Check sheet for the modelled part. Datum: model origin and axes. Units: mm. Round coordinates to 2 decimals unless told otherwise and drop trailing zeros. Write each loop counter-clockwise with the first axis right and the second up, starting at its lowest first coordinate (ties: lowest second). Pieces come first, ordered by that corner, then holes.
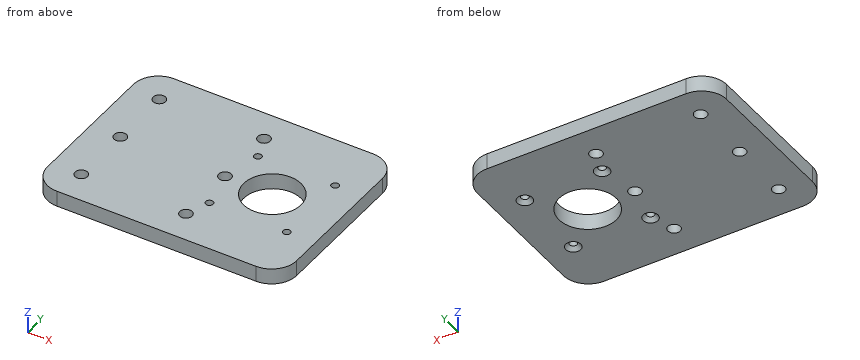
from build123d import *

# Parameters (mm, degrees)
SKETCH1_W             = 100
SKETCH1_H             = 75
PLATE_DEPTH           = 6.35
SKETCH2_R             = 2.5
CUT_IDLER_HOLES_DEPTH = 126.161186076
SKETCH3_R             = 1.5
SKETCH3_R_2           = 11.5
CUT_MOTOR_HOLES_DEPTH = 126.161186076
CHAMFER1_SIZE         = 1.5
FILLET1_R             = 10


with BuildPart() as part:
    # Sketch1 → plate (new body)
    with BuildSketch(Plane.XY):
        with Locations((50, 37.5)):
            Rectangle(SKETCH1_W, SKETCH1_H)
    extrude(amount=PLATE_DEPTH)

    # Sketch2 → cut idler holes (cut, through all)
    with BuildSketch(Plane.XY.offset(6.35)):
        with Locations((12, 62.5)):
            Circle(SKETCH2_R)
        with Locations((12, 12.5)):
            Circle(SKETCH2_R)
        with Locations((54, 37.5)):
            Circle(SKETCH2_R)
        with Locations((54, 62.5)):
            Circle(SKETCH2_R)
        with Locations((12, 37.5)):
            Circle(SKETCH2_R)
        with Locations((54, 12.5)):
            Circle(SKETCH2_R)
    extrude(amount=-CUT_IDLER_HOLES_DEPTH, mode=Mode.SUBTRACT)

    # Sketch3 → cut motor holes (cut, through all)
    with BuildSketch(Plane.XY.offset(6.35)):
        with Locations((57.5, 53)):
            Circle(SKETCH3_R)
        with Locations((88.5, 53)):
            Circle(SKETCH3_R)
        with Locations((88.5, 22)):
            Circle(SKETCH3_R)
        with Locations((57.5, 22)):
            Circle(SKETCH3_R)
        with Locations((73, 37.5)):
            Circle(SKETCH3_R_2)
    extrude(amount=-CUT_MOTOR_HOLES_DEPTH, mode=Mode.SUBTRACT)

    # Chamfer1
    chamfer1_edges = [part.edges().sort_by_distance(p)[0] for p in [
        (56, 53, 0),
        (87, 22, 0),
        (56, 22, 0),
        (87, 53, 0),
    ]]
    chamfer(chamfer1_edges, length=CHAMFER1_SIZE)

    # Fillet1
    fillet1_edges = [part.edges().sort_by_distance(p)[0] for p in [
        (0, 75, 3.175),
        (100, 75, 3.175),
        (100, 0, 3.175),
        (0, 0, 3.175),
    ]]
    fillet(fillet1_edges, radius=FILLET1_R)


solid = part.part
1. Go/stop test with a flat-tipped pin: pin 1 (4 mm diameter, centred on x = 57.5, y = 53, fed in from -Z). Record where the tip stops, or that it passes through.
2. Sectioned sample at A-A, the plane y = 37.5. Enter the section's corners in (x, z), plus the area to 3 significant figures.
3. Sectioned sample at C-C, the plane z = 2.5. Give the number of separate pieces and of enclosed holes in the cut face, plus the area to 3 significant figures.
4. Sectioned sample at D-D, the plane y = 12.5. Enter the section's corners in (x, z).
5. Scan lines: line 1 along Y through (x, z) = (12, 5); line 2 along X through (y, z) = (21.5, 6.25); line 3 along X through (y, z) = (29.5, 1). Record each from-to range of solid material in increasing order.
6. Sectioned sample at B-B, the plane y = 22. Enter the section's corners in (x, z), plus the area to 3 significant figures.
Computed values:
1. pin 1: stops at z = 1
2. outline: (0, 0) - (9.5, 0) - (9.5, 6.35) - (0, 6.35) - close; (14.5, 0) - (51.5, 0) - (51.5, 6.35) - (14.5, 6.35) - close; (56.5, 0) - (61.5, 0) - (61.5, 6.35) - (56.5, 6.35) - close; (84.5, 0) - (100, 0) - (100, 6.35) - (84.5, 6.35) - close
2. area: 425 mm2
3. separate pieces: 1
3. enclosed holes: 11
3. area: 6,850 mm2
4. outline: (0, 0) - (9.5, 0) - (9.5, 6.35) - (0, 6.35) - close; (14.5, 0) - (51.5, 0) - (51.5, 6.35) - (14.5, 6.35) - close; (56.5, 0) - (100, 0) - (100, 6.35) - (56.5, 6.35) - close
5. line 1: y = 0 to 10, 15 to 35, 40 to 60, 65 to 75
5. line 2: x = 0 to 56.09, 58.91 to 87.09, 89.91 to 100
5. line 3: x = 0 to 64.74, 81.26 to 100
6. outline: (0, 0) - (54.5, 0) - (56, 1.5) - (56, 6.35) - (0, 6.35) - close; (59, 1.5) - (60.5, 0) - (85.5, 0) - (87, 1.5) - (87, 6.35) - (59, 6.35) - close; (90, 1.5) - (91.5, 0) - (100, 0) - (100, 6.35) - (90, 6.35) - close
6. area: 592 mm2
